from build123d import *

# Parameters (mm, degrees)
F0_W      = 98.425
F0_H      = 19.05
F1_DEPTH  = 98.425
F2_W      = 123.825
F2_H      = 50.8
F3_DEPTH  = 42.545
F5_W      = 9.525
F5_H      = 25.4
F6_DEPTH  = 15.875
F8_DEPTH  = 123.826
F9_W      = 9.525
F9_H      = 25.4
F10_DEPTH = 15.875
F12_DEPTH = 98.426
F13_W     = 31.75
F13_H     = 9.525
F14_DEPTH = 98.425
F15_DEPTH = 123.826
F16_R     = 9.525
F17_DEPTH = 28.576


with BuildPart() as f1:
    # F0 (on Front) → F1 (new body)
    with BuildSketch(Plane.XZ):
        with Locations((-42.737771, 20.002501)):
            Rectangle(F0_W, F0_H)
    extrude(amount=F1_DEPTH)

    # F2 (on face) → F3 (join)
    with BuildSketch(Plane.XY.offset(29.527501)):
        with Locations((-30.037771, -25.4)):
            Rectangle(F2_W, F2_H)
    extrude(amount=F3_DEPTH)

    # F5 (on face) → F6 (join)
    with BuildSketch(Plane.XZ.offset(50.8)):
        with Locations((-87.187771, 42.227501)):
            Rectangle(F5_W, F5_H)
    extrude(amount=F6_DEPTH)

    # F7 (on face) → F8 (cut, through all)
    with BuildSketch(Plane(origin=(-91.950271, 0, 0), x_dir=(0, -1, 0), z_dir=(-1, 0, 0))):
        Polygon((66.675, 54.927501), (50.8, 54.927501), (66.675, 29.527501), align=None)
    extrude(amount=-F8_DEPTH, mode=Mode.SUBTRACT)

    # F9 (on face) → F10 (join)
    with BuildSketch(Plane.XZ.offset(50.8)):
        with Locations((1.712229, 42.227501)):
            Rectangle(F9_W, F9_H)
    extrude(amount=F10_DEPTH)

    # F11 (on face) → F12 (cut, through all)
    with BuildSketch(Plane.YZ.offset(6.474729)):
        Polygon((-66.675, 29.527501), (-50.8, 54.927501), (-66.675, 54.927501), align=None)
    extrude(amount=-F12_DEPTH, mode=Mode.SUBTRACT)

    # F13 (on face) → F14 (join)
    with BuildSketch(Plane.YZ.offset(6.474729)):
        with Locations((-73.025, 5.715001)):
            Rectangle(F13_W, F13_H)
    extrude(amount=-F14_DEPTH)

    # F4 (on face) → F15 (cut, through all)
    with BuildSketch(Plane(origin=(-91.950271, 0, 0), x_dir=(0, -1, 0), z_dir=(-1, 0, 0))):
        Polygon((33.3375, 72.072501), (17.4625, 72.072501), (17.4625, 62.547501), (11.065112, 62.547501), (11.065112, 54.610001), (42.815112, 54.610001), (42.815112, 62.547501), (33.3375, 62.547501), align=None)
    extrude(amount=-F15_DEPTH, mode=Mode.SUBTRACT)

    # F16 (on face) → F17 (cut, through all)
    with BuildSketch(Plane.XY.offset(29.527501)):
        with Locations((-42.737771, -73.025)):
            Circle(F16_R)
    extrude(amount=-F17_DEPTH, mode=Mode.SUBTRACT)


solid = f1.part
Verification items for the finished model (mm, model axes). A direction names the side the tool comes from. Round coordinates to 2 decimals unless told otherwise and drop trailing zeros. Loops run counter-clockwise (first coordinate to the right, second up) from the corner with the lowest first, then second, coordinate; pieces in that order, holes last. Notation, with made-up numbers: (38, -10.5) - (54, -10.5) arc R32 cw to (54, 23.5) - close; hole circle Ø6 at (49.5, 40.25). An arc over 180 degrees is marked (long way). Use a Markdown table: item, result. Add a question column.
1. Thickness scan on probe 1 along Y at (x, z) = (-0.5, 67.5); probe 2 along Y at (x, z) = (-78.5, 58); probe 3 along X at (y, z) = (-55.5, 18.5). Record the ranges inside material, lowest first. Write a range as [from, to].
2. Release check for a two-part mould opening along Y. For faces 1 (the face through (6.475, -49, 22)), 2 (the face through (1.78, -58.85, 42.05)), 3 (the face through (-31, -14, 62.548)) record: released by +Y, released by -Y, zero draft, split by the parting line, or undercut.
3. Section check A-A, the plane y = -80.5. Record the boundary of the cut face in (x, z).
4. Access from +Z, -Z, +X, -X, +Y, -Y to the whole of each face (thin tool, end or side, straight path). Record for faces 4 (the face through (-31, -17.462, 67)), 5 (the face through (-82.425, -57, 39)), 6 (the face through (-42, -57.15, 6)), 7 (the face through (-31, -42.815, 59)), 8 (the face through (-43, -94, 10.478)).
5. Section check D-D, the plane y = -8.5. Record the boundary of the cut face in (x, z).
6. Gauge pin test, flat ends, axial feed: pin 1 (3 mm diameter, centred on x = -65.5, z = 3.5, fed in from +Y); pin 2 (17.5 mm diameter, centred on y = -59, z = 45, fed in from -X); pin 3 (1 mm diameter, centred on x = -19.5, y = -49, fed in from -Z); pin 4 (3 mm diameter, centred on y = -56, z = 9, fed in from +X). Record the tip position at first contact, or that the pin passes through.
Checks:
| question | item | result |
|---|---|---|
| 1 | probe 1 | y = [-50.8, -33.34], [-17.46, 0] |
| 1 | probe 2 | y = [-50.8, -42.82], [-11.07, 0] |
| 1 | probe 3 | x = [-91.95, 6.47] |
| 2 | face 1 | zero draft |
| 2 | face 2 | released by -Y |
| 2 | face 3 | undercut |
| 3 | outline | (-91.95, 0.95) - (-48.64, 0.95) - (-48.64, 29.53) - (-91.95, 29.53) - close; (-36.83, 0.95) - (6.47, 0.95) - (6.47, 29.53) - (-36.83, 29.53) - close |
| 4 | face 4 | +Z, +X, -X |
| 4 | face 5 | +Z, -Y |
| 4 | face 6 | -Z, +X, -X, +Y |
| 4 | face 7 | +X, -X |
| 4 | face 8 | -Z, +X, -X, -Y |
| 5 | outline | (-91.95, 10.48) - (6.47, 10.48) - (6.47, 29.53) - (31.87, 29.53) - (31.87, 72.07) - (-91.95, 72.07) - close |
| 6 | pin 1 | stops at y = -57.15 |
| 6 | pin 2 | stops at x = -91.95 |
| 6 | pin 3 | stops at z = 10.48 |
| 6 | pin 4 | stops at x = 6.47 |
